Build history of the part. All positions in model axes, mm. Give positions to 0.01 mm unless a question says otherwise; leave off trailing zeros. Order: outer loops, then holes, each group sorted by start corner. A loop starts at its lowest first (then second) coordinate and runs counter-clockwise, first axis right, second up. Notation, with made-up numbers: (-36, 48.25) - (12, 48.25) arc R24 ccw to (12, 85.25) - close; hole circle Ø4 at (24.5, 54.5). An arc over 180 degrees is marked (long way). Use a Markdown table: item, result. Add a question column.
(1) Flat gauge pins, fed straight in: pin 1 (9.5 mm diameter, centred on x = -71.5, y = 0, fed in from +Z); pin 2 (2.5 mm diameter, centred on y = -80, z = 5.5, fed in from -X); pin 3 (2.5 mm diameter, centred on y = -79.5, z = 7, fed in from +X); pin 4 (2 mm diameter, centred on y = -46, z = 16, fed in from +X). Where does each tip first touch, or does it go through?
(2) Slice it at B-B (y = 0). Count the separate pieces of the cut face and the enclosed holes in it, then the cut area to 3 significant figures.
(3) Slice it at A-A (z = 4.25). Write the cut outline in (x, y).
(4) Wall check: line 1 (Y direction, x = 5, z = 7.25) (3 decimals); line 2 (Y direction, x = 65, z = 16.5); line 3 (X direction, y = -27.5, z = 5.75). Give the ranges that are in metal, low to high.
from build123d import *

# Parameters (mm, degrees)
F0_R     = 8
F1_DEPTH = 20
F2_R     = 3
F3_R     = 1


with BuildPart() as f1:
    # F0 (on Top) → F1 (new body)
    with BuildSketch(Plane.XY):
        with BuildLine():
            Line((-43.5, -85), (0, -85))
            Line((0, -85), (43.5, -85))
            Line((43.5, -85), (43.5, -76.764249))
            ThreePointArc((43.5, -76.764249), (46.591944, -66.081663), (54.911765, -58.702073))
            ThreePointArc((54.911765, -58.702073), (91.61519, -7.06238), (66.93343, 51.286657))
            ThreePointArc((66.93343, 51.286657), (49.963072, 71.157412), (42.189443, 96.105572))
            Line((42.189443, 96.105572), (37, 148))
            ThreePointArc((37, 148), (26.594735, 184.193845), (4.090054, 214.389927))
            ThreePointArc((4.090054, 214.389927), (0, 216), (-4.090054, 214.389927))
            ThreePointArc((-4.090054, 214.389927), (-26.594735, 184.193845), (-37, 148))
            Line((-37, 148), (-42.189443, 96.105572))
            ThreePointArc((-42.189443, 96.105572), (-49.963072, 71.157412), (-66.93343, 51.286657))
            ThreePointArc((-66.93343, 51.286657), (-91.61519, -7.06238), (-54.911765, -58.702073))
            ThreePointArc((-54.911765, -58.702073), (-46.591944, -66.081663), (-43.5, -76.764249))
            Line((-43.5, -76.764249), (-43.5, -85))
        make_face()
        with Locations((-71.5, 0)):
            Circle(F0_R, mode=Mode.SUBTRACT)
        with Locations((71.5, 0)):
            Circle(F0_R, mode=Mode.SUBTRACT)
        with Locations((0, 194)):
            Circle(F0_R, mode=Mode.SUBTRACT)
    extrude(amount=F1_DEPTH)

    # F2
    f2_edges = [f1.edges().sort_by_distance(p)[0] for p in [
        (39.594721, 122.052786, 20),
    ]]
    fillet(f2_edges, radius=F2_R)

    # F3
    f3_edges = [f1.edges().sort_by_distance(p)[0] for p in [
        (-8, 194, 20),
        (-79.5, 0, 20),
        (63.5, 0, 20),
    ]]
    fillet(f3_edges, radius=F3_R)


solid = f1.part
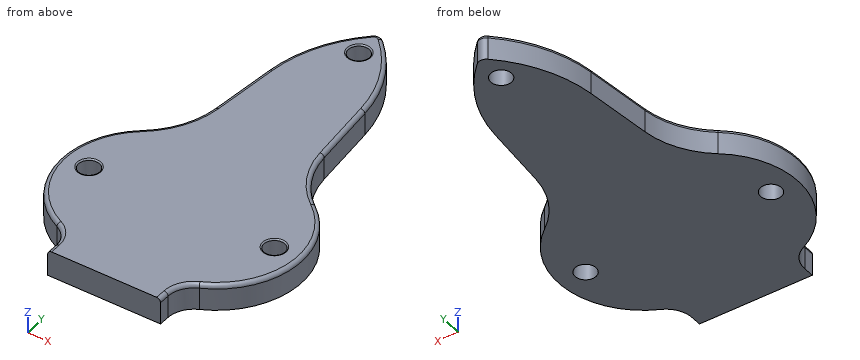
Solution:
| question | item | result |
|---|---|---|
| 1 | pin 1 | through |
| 1 | pin 2 | x = -43.5 |
| 1 | pin 3 | x = 43.5 |
| 1 | pin 4 | x = 73.9 |
| 2 | separate pieces | 3 |
| 2 | enclosed holes | 0 |
| 2 | area | 3,040 mm2 |
| 3 | outline | (-66.93, 51.29) arc R65 ccw to (-54.91, -58.7) arc R20 cw to (-43.5, -76.76) - (-43.5, -85) - (43.5, -85) - (43.5, -76.76) arc R20 cw to (54.91, -58.7) arc R65 ccw to (66.93, 51.29) arc R65 cw to (42.19, 96.11) - (37, 148) arc R105.02 ccw to (4.09, 214.39) arc R6 ccw to (-4.09, 214.39) arc R105.02 ccw to (-37, 148) - (-42.19, 96.11) arc R65 cw to start; hole circle Ø16 at (-71.5, 0); hole circle Ø16 at (0, 194); hole circle Ø16 at (71.5, 0) |
| 4 | line 1 | -85 to 187.755, 200.245 to 213.532 |
| 4 | line 2 | -52.74 to -4.66, 4.66 to 52.85 |
| 4 | line 3 | -85.9 to 85.9 |
